```python
from build123d import *

# Parameters (mm, degrees)
SKETCH1_W               = 34
SKETCH1_H               = 19
BOSS_EXTRUDE1_DEPTH     = 20.2
SKETCH2_OUTSIDE_W       = 47.224
SKETCH2_OUTSIDE_H       = 32.224
SKETCH2_OUTSIDE_W_2     = 32.9
SKETCH2_OUTSIDE_H_2     = 18.5
CUT_EXTRUDE2_DEPTH      = 44.462627624
CUT_EXTRUDE8_DEPTH      = 36.679686097
CUT_EXTRUDE8_DEPTH_BACK = 36.679686097
SKETCH3_W               = 0.125
SKETCH3_H               = 9
CUT_EXTRUDE3_DEPTH      = 23.6
CHAMFER1_SIZE           = 1
CHAMFER2_SIZE           = 1
CHAMFER3_SIZE           = 1
CHAMFER4_SIZE           = 1
SKETCH10_R              = 3
BOSS_EXTRUDE3_DEPTH     = 3
FILLET1_R               = 2
TAP1_D                  = 3.242
TAP1_DEPTH              = 6
TAP1_TIP                = 0.973995063


with BuildPart() as part:
    # Sketch1 → Boss-Extrude1 (new, symmetric)
    with BuildSketch(Plane(origin=(0, 0, 0), x_dir=(0, 0, -1), z_dir=(1, 0, 0))):
        with Locations((0, 14.5)):
            Rectangle(SKETCH1_W, SKETCH1_H)
    extrude(amount=BOSS_EXTRUDE1_DEPTH, both=True)

    # Sketch2 outside → Cut-Extrude2 (cut, through all)
    with BuildSketch(Plane(origin=(11.8, 0, 0), x_dir=(0, 0, -1), z_dir=(1, 0, 0))):
        with Locations((0, 14.5)):
            Rectangle(SKETCH2_OUTSIDE_W, SKETCH2_OUTSIDE_H)
        with Locations((0, 14.25)):
            Rectangle(SKETCH2_OUTSIDE_W_2, SKETCH2_OUTSIDE_H_2, mode=Mode.SUBTRACT)
    cut_extrude2 = extrude(amount=CUT_EXTRUDE2_DEPTH, mode=Mode.SUBTRACT)

    # Mirror1: Cut-Extrude2 across plane
    add(cut_extrude2.mirror(Plane(origin=(0, 0, 0), x_dir=(0, 0, 1), z_dir=(1, 0, 0))), mode=Mode.SUBTRACT)

    # Sketch5 → Cut-Extrude8 (cut, two sides: drawn at the far end of the back side and taken through both)
    with BuildSketch(Plane(origin=(0, 0, 0), x_dir=(0, 0, -1), z_dir=(1, 0, 0)).offset(-CUT_EXTRUDE8_DEPTH_BACK)):
        with BuildLine():
            Line((-5.692330317, 12.5), (5.692330317, 12.5))
            Line((5.692330317, 12.5), (6.192330317, 12))
            ThreePointArc((6.192330317, 12), (6.706274607, 11.346743741), (7.5, 11.1))
            Line((7.5, 11.1), (7.5, 9.5))
            ThreePointArc((7.5, 9.5), (6.1, 8.1), (7.5, 6.7))
            Line((7.5, 6.7), (7.5, 1))
            Line((7.5, 1), (6.5, 0))
            Line((6.5, 0), (-6.5, 0))
            Line((-6.5, 0), (-7.5, 1))
            Line((-7.5, 1), (-7.5, 6.7))
            ThreePointArc((-7.5, 6.7), (-6.1, 8.1), (-7.5, 9.5))
            Line((-7.5, 9.5), (-7.5, 11.1))
            ThreePointArc((-7.5, 11.1), (-6.706274607, 11.346743741), (-6.192330317, 12))
            Line((-6.192330317, 12), (-5.692330317, 12.5))
        make_face()
    extrude(amount=CUT_EXTRUDE8_DEPTH + CUT_EXTRUDE8_DEPTH_BACK, mode=Mode.SUBTRACT)

    # Sketch3 → Cut-Extrude3 (cut)
    with BuildSketch(Plane(origin=(11.8, 0, 0), x_dir=(0, 0, -1), z_dir=(1, 0, 0))):
        with Locations((-16.9375, 9.5)):
            Rectangle(SKETCH3_W, SKETCH3_H)
    cut_extrude3 = extrude(amount=-CUT_EXTRUDE3_DEPTH, mode=Mode.SUBTRACT)

    # Mirror2: Cut-Extrude3 across plane
    add(cut_extrude3.mirror(Plane.XY), mode=Mode.SUBTRACT)

    # Chamfer1
    chamfer1_edges = [part.edges().sort_by_distance(p)[0] for p in [
        (16, 23.5, -16.45),
        (16, 23.5, 16.45),
        (-16, 23.5, 16.45),
        (-16, 23.5, -16.45),
    ]]
    chamfer(chamfer1_edges, length=CHAMFER1_SIZE)

    # Chamfer2
    chamfer2_edges = [part.edges().sort_by_distance(p)[0] for p in [
        (0, 24, 17),
        (0, 24, -17),
    ]]
    chamfer(chamfer2_edges, length=CHAMFER2_SIZE)

    # Chamfer3
    chamfer3_edges = [part.edges().sort_by_distance(p)[0] for p in [
        (16, 5, 16.45),
        (16, 5, -16.45),
        (-16, 5, -16.45),
        (-16, 5, 16.45),
    ]]
    chamfer(chamfer3_edges, length=CHAMFER3_SIZE)

    # Chamfer4
    chamfer4_edges = [part.edges().sort_by_distance(p)[0] for p in [
        (0, 5, 16.875),
        (0, 5, -16.875),
    ]]
    chamfer(chamfer4_edges, length=CHAMFER4_SIZE)

    # Sketch10 → Boss-Extrude3 (add)
    with BuildSketch(Plane(origin=(20.2, 0, 0), x_dir=(0, 0, -1), z_dir=(1, 0, 0))):
        with Locations((0, 18)):
            Circle(SKETCH10_R)
    extrude(amount=BOSS_EXTRUDE3_DEPTH)

    # Fillet1
    fillet1_edges = [part.edges().sort_by_distance(p)[0] for p in [
        (23.2, 18, 3),
    ]]
    fillet(fillet1_edges, radius=FILLET1_R)

    # Tap1
    with Locations(Plane(origin=(0, 24, 0), x_dir=(1, 0, 0), z_dir=(0, 1, 0))):
        with Locations((0, -13), (0, 13)):
            Hole(TAP1_D / 2, depth=TAP1_DEPTH)
            with Locations((0, 0, -(TAP1_DEPTH + TAP1_TIP / 2))):  # 118° drill point
                Cone(0, TAP1_D / 2, TAP1_TIP, mode=Mode.SUBTRACT)


solid = part.part
```
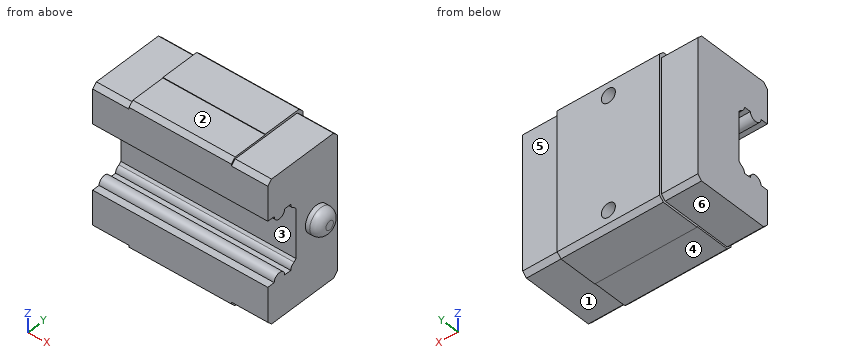
Geometry: final body of the model. Coordinates: model frame, mm. Face numbers are marked on the shaded views. A direction names the side the tool comes from. Give positions to 0.01 mm unless a question says otherwise; leave off trailing zeros. Loops run counter-clockwise (first coordinate to the right, second up) from the corner with the lowest first, then second, coordinate; pieces in that order, holes last. Notation, with made-up numbers: (46.25, 87) -> (95.25, 87) arc R25 ccw to (95.25, 107) -> close; hole circle Ø3 at (-35, 11.5). An arc over 180 degrees is marked (long way). Use one line per item in the form item = value.
Item 1: Section query D-D on y = 22. Output: boundary loops of the cut face in (x, z).
A:
outline = (-20.2, -16.45) -> (-11.8, -16.45) -> (-11.8, -17) -> (11.8, -17) -> (11.8, -16.45) -> (20.2, -16.45) -> (20.2, 16.45) -> (11.8, 16.45) -> (11.8, 17) -> (-11.8, 17) -> (-11.8, 16.45) -> (-20.2, 16.45) -> close; hole circle Ø3.24 at (0, -13); hole circle Ø3.24 at (0, 13)
Item 2: Access query for the marked faces 4, 5 and 6. Directions: +Z, -Z, +X, -X, +Y, -Y. A direction counts if a zero-diameter tool reaches every point of the face in a straight line with its end or side. Return the directions, or none.
A:
face_4 = -Z, +X, -X, -Y
face_5 = +Z, -Z, +X, +Y
face_6 = -Z, -X, +Y, -Y
Item 3: Section query C-C on x = 17. Output: boundary loops of the cut face in (y, z), and give its area (3 significant figures).
A:
outline = (5, -15.45) -> (6, -16.45) -> (22.5, -16.45) -> (23.5, -15.45) -> (23.5, 15.45) -> (22.5, 16.45) -> (6, 16.45) -> (5, 15.45) -> (5, 7.5) -> (6.7, 7.5) arc R1.4 ccw to (9.5, 7.5) -> (11.1, 7.5) arc R1.4 ccw to (12, 6.19) -> (12.5, 5.69) -> (12.5, -5.69) -> (12, -6.19) arc R1.4 ccw to (11.1, -7.5) -> (9.5, -7.5) arc R1.4 ccw to (6.7, -7.5) -> (5, -7.5) -> close
area = 504 mm^2
Item 4: Section query A-A on y = 7.25. Output: boundary loops of the cut face in (x, z) (3 decimals), and give its area (3 significant figures).
A:
outline = (-20.2, -16.45) -> (-11.8, -16.45) -> (-11.8, -16.875) -> (11.8, -16.875) -> (11.8, -16.45) -> (20.2, -16.45) -> (20.2, -6.388) -> (-20.2, -6.388) -> close; (-20.2, 6.388) -> (20.2, 6.388) -> (20.2, 16.45) -> (11.8, 16.45) -> (11.8, 16.875) -> (-11.8, 16.875) -> (-11.8, 16.45) -> (-20.2, 16.45) -> close
area = 833 mm^2
Item 5: Pin query (flat end, axial travel): P1, Ø6.5, axis at x = -4, y = 12, coming from the +Z side; P2, Ø1.8, axis at x = 0, y = 10, coming from the +Z side (3 decimals); P3, Ø0.5, axis at x = 4.5, y = 5.5, coming from the -Z side (3 decimals); P4, Ø3, axis at x = -13.5, z = -3.5, coming from the +Y side. Return the tip coordinate at first contact, or that it passes through.
A:
P1 = 17
P2 = 16.875
P3 = -16.625
P4 = 23.5
Item 6: Section query B-B on z = -8. Output: boundary loops of the cut face in (x, y).
A:
outline = (-20.2, 5) -> (20.2, 5) -> (20.2, 23.5) -> (11.8, 23.5) -> (11.8, 24) -> (-11.8, 24) -> (-11.8, 23.5) -> (-20.2, 23.5) -> close
Item 7: Draft query along Z for the marked faces 1, 2 and 3. Return one class per face: pulls with the +Z half, pulls with the -Z half, needs draft (parallel to the pull), parting line crosses it, or undercut.
A:
face_1 = pulls with the -Z half
face_2 = pulls with the +Z half
face_3 = undercut
Item 8: Line query: probe 1 along Z at (x, y) = (0, 19.9); probe 2 along X at (y, z) = (21.3, 13); probe 3 along X at (y, z) = (17, 8.5). Output: solid intervals per line, ascending.
A:
probe_1 = -17 to -14.62, -11.38 to 11.38, 14.62 to 17
probe_2 = -20.2 to -1.62, 1.62 to 20.2
probe_3 = -20.2 to 20.2
